Verification items for the finished model (mm, model axes). A direction names the side the tool comes from. Round coordinates to 2 decimals unless told otherwise and drop trailing zeros. Order: outer loops, then holes, each group sorted by start corner. A loop starts at its lowest first (then second) coordinate and runs counter-clockwise, first axis right, second up. Notation, with made-up numbers: (-26.5, 2.25) -> (-8.5, 2.25) arc R21 cw to (-8.5, 12.25) -> close; hole circle Ø4 at (0, -6). An arc over 180 degrees is marked (long way). Return JSON: item names as keys, results as strings. Group by question number.
Item 1: Sectioned sample at C-C on x = -7.5. Record the cut outline in (y, z), plus the area to 3 significant figures.
Item 2: Depth check by flat-ended pin: pin 1 Ø1 at (x, z) = (23, -18.5) entering from -Y; pin 2 Ø10 at (x, z) = (-15.5, -1) entering from -Y; pin 3 Ø19.5 at (x, z) = (-23.5, -2) entering from +Y. Enter the tip coordinate at first touch or a pass-through.
Item 3: Scan lines: probe 1 along Z at (x, y) = (-29, -11.5); probe 2 along X at (y, z) = (20.5, 6); probe 3 along Z at (x, y) = (-35, 22.5). Record each from-to range of solid material in increasing order. Write a range as from..to.
Item 4: Sectioned sample at D-D on y = -13. Record the cut outline in (x, z), plus the area to 3 significant figures.
Item 5: Sectioned sample at A-A on z = 2.5. Record the cut outline in (x, y), plus the area to 3 significant figures.
Item 6: Sectioned sample at B-B on y = 36.5. Record the cut outline in (x, z), plus the area to 3 significant figures.
Item 7: Access from +Z, -Z, +X, -X, +Y, -Y to the whole of each face (thin tool, end or side, straight path). Record for faces 1 (the flat face through (22, -8, -18.753)), 2 (the flat face through (-8, 30.699, 0)), 3 (the flat face through (-51.461, 23, 0)), 4 (the flat face through (-27, 24, 12.576)).
Item 8: Draft check along X on faces 5 (the flat face through (-8, 47.488, 0)), 6 (the flat face through (-27, 24, -11.922)), 7 (the flat face through (41.792, 15, 0)), 8 (the flat face through (-14.185, 24, 0)). Enter one of: pulls with the +X half, pulls with the -X half, needs draft (parallel to the pull), parting line crosses it, or undercut.
```python
from build123d import *

# Parameters (mm, degrees)
F1_DEPTH  = 18.753305
F3_DEPTH  = 15.54585
F5_W      = 37.2849525884
F5_H      = 18.1331187487
F6_DEPTH  = 53.05346
F7_W      = 16.7898200452
F7_H      = 29.3058659881
F8_DEPTH  = 55.0196293017
F9_R      = 3.2034431946
F10_DEPTH = 25
F11_R     = 3.2034431946
F13_DEPTH = 3.90451
F13_TAPER = 10
F14_W     = 25.0537479296
F14_H     = 24.4980249554
F18_DEPTH = 12.2033338994
F16_R     = 2.0640703288
F17_DEPTH = 34.12419


with BuildPart() as f1:
    # F0 (on Top) → F1 (new body, symmetric)
    with BuildSketch(Plane.XY):
        Polygon((-5.5769230239, 51.2194294688), (-51.4608863181, 51.2194294688), (-51.4608863181, 4.5192311518), (-5.5769230239, 4.5192311518), (41.7920313589, 4.5192311518), (41.7920313589, 25.2884626389), (-5.5769230239, 25.2884626389), align=None)
    extrude(amount=F1_DEPTH, both=True)

    # F2 (on face) → F3 (join)
    with BuildSketch(Plane.XY.offset(18.753305)):
        with BuildLine():
            ThreePointArc((-51.4608863181, 23.7576867202), (-46.417709158, -17.9074521958), (-10.9429109093, 4.5192311518))
            Line((-10.9429109093, 4.5192311518), (-51.4608863181, 4.5192311518))
            Line((-51.4608863181, 4.5192311518), (-51.4608863181, 23.7576867202))
        make_face()
        with BuildLine():
            Line((-51.4608863181, 4.5192311518), (-10.9429109093, 4.5192311518))
            ThreePointArc((-10.9429109093, 4.5192311518), (-25.1207540769, 26.9459144993), (-51.4608863181, 23.7576867202))
            Line((-51.4608863181, 23.7576867202), (-51.4608863181, 4.5192311518))
        make_face()
        with BuildLine():
            ThreePointArc((32.7010839123, 4.5192311518), (22.6923078299, 8.5573695546), (12.6835317475, 4.5192311518))
            Line((12.6835317475, 4.5192311518), (32.7010839123, 4.5192311518))
        make_face()
        with BuildLine():
            Line((32.7010839123, 4.5192311518), (12.6835317475, 4.5192311518))
            ThreePointArc((12.6835317475, 4.5192311518), (17.0504227911, -19.1388547133), (37.1150626747, -5.8653852902))
            ThreePointArc((37.1150626747, -5.8653852902), (35.9657772529, -0.2235002514), (32.7010839123, 4.5192311518))
        make_face()
    extrude(amount=F3_DEPTH)

    # F4: F1 across plane


with BuildPart() as f1_1:
    add(f1.part)
    add(f1.part.mirror(Plane.XY))

    # F5 (on face) → F6 (cut, through all)
    with BuildSketch(Plane.XY.offset(18.753305)):
        with Locations((-28.6624371074, 39.2740033567)):
            Rectangle(F5_W, F5_H)
    extrude(amount=-F6_DEPTH, mode=Mode.SUBTRACT)

    # F7 (on face) → F8 (cut, through all)
    with BuildSketch(Plane.YZ.offset(-5.5769230239)):
        with Locations((39.0934366733, 0.1526279375)):
            Rectangle(F7_W, F7_H)
    extrude(amount=-F8_DEPTH, mode=Mode.SUBTRACT)

    # F9 (on face) → F10 (join)
    with BuildSketch(Plane(origin=(0, 25.2884626389, 0), x_dir=(-1, 0, 0), z_dir=(0, 1, 0))):
        with Locations((-18.5051690787, 10.1850191131)):
            Circle(F9_R)
    extrude(amount=F10_DEPTH)

    # F11 (on face) → F13 (join)
    with BuildSketch(Plane(origin=(0, 50.2884626389, 0), x_dir=(-1, 0, 0), z_dir=(0, 1, 0))):
        with Locations((-18.5051690787, 10.1850191131)):
            Circle(F11_R)
    extrude(amount=F13_DEPTH, taper=F13_TAPER)

    # F14 (on face) → F18 (cut)
    with BuildSketch(Plane(origin=(0, 30.2074439824, 0), x_dir=(-1, 0, 0), z_dir=(0, 1, 0))):
        with Locations((26.7121638171, 0.3265431151)):
            Rectangle(F14_W, F14_H)
    extrude(amount=-F18_DEPTH, mode=Mode.SUBTRACT)

    # F16 (on face) → F17 (cut)
    with BuildSketch(Plane(origin=(0, 54.1929726389, 0), x_dir=(-1, 0, 0), z_dir=(0, 1, 0))):
        with Locations((-18.574340269, 10.1817082614)):
            Circle(F16_R)
    extrude(amount=-F17_DEPTH, mode=Mode.SUBTRACT)


solid = f1_1.part
```
Recorded:
{
 "1": {"outline": "(4.52, -18.75) -> (51.22, -18.75) -> (51.22, 18.75) -> (4.52, 18.75) -> close; hole (30.7, -14.5) -> (47.49, -14.5) -> (47.49, 14.81) -> (30.7, 14.81) -> close", "area": "1,260 mm²"},
 "2": {"pin 1": "y = -20.29", "pin 2": "y = 4.52", "pin 3": "y = 51.22"},
 "3": {"probe 1": "-34.3..-18.75, 18.75..34.3", "probe 2": "-51.46..-39.24, -14.19..41.79", "probe 3": "-34.3..-11.92, 12.58..34.3"},
 "4": {"outline": "(-53.36, -34.3) -> (-18.18, -34.3) -> (-18.18, -18.75) -> (-53.36, -18.75) -> close; (-53.36, 18.75) -> (-18.18, 18.75) -> (-18.18, 34.3) -> (-53.36, 34.3) -> close; (10.16, -34.3) -> (35.23, -34.3) -> (35.23, -18.75) -> (10.16, -18.75) -> close; (10.16, 18.75) -> (35.23, 18.75) -> (35.23, 34.3) -> (10.16, 34.3) -> close", "area": "1,870 mm²"},
 "5": {"outline": "(-51.46, 4.52) -> (41.79, 4.52) -> (41.79, 25.29) -> (-5.58, 25.29) -> (-5.58, 30.7) -> (-10.02, 30.7) -> (-10.02, 30.21) -> (-14.19, 30.21) -> (-14.19, 18) -> (-39.24, 18) -> (-39.24, 30.21) -> (-47.3, 30.21) -> (-47.3, 30.7) -> (-51.46, 30.7) -> close; (-51.46, 47.49) -> (-47.3, 47.49) -> (-47.3, 48.34) -> (-10.02, 48.34) -> (-10.02, 47.49) -> (-5.58, 47.49) -> (-5.58, 51.22) -> (-51.46, 51.22) -> close", "area": "2,000 mm²"},
 "6": {"outline": "(-51.46, -18.75) -> (-47.3, -18.75) -> (-47.3, -14.5) -> (-51.46, -14.5) -> close; (-51.46, 14.81) -> (-47.3, 14.81) -> (-47.3, 18.75) -> (-51.46, 18.75) -> close; (-10.02, -18.75) -> (-5.58, -18.75) -> (-5.58, -14.5) -> (-10.02, -14.5) -> close; (-10.02, 14.81) -> (-5.58, 14.81) -> (-5.58, 18.75) -> (-10.02, 18.75) -> close; circle Ø6.41 at (18.51, 10.19); hole circle Ø4.13 at (18.57, 10.18)", "area": "89.4 mm²"},
 "7": {"face 1": "+X, -X, -Y", "face 2": "-X", "face 3": "-X, +Y, -Y", "face 4": "none"},
 "8": {"face 5": "needs draft", "face 6": "undercut", "face 7": "pulls with the +X half", "face 8": "undercut"}
}
